The listing builds one solid part. Answer for the finished solid, in the listing's coordinates (mm). Face numbers are marked on the shaded views. Round coordinates to 2 decimals unless told otherwise and drop trailing zeros. Write each loop counter-clockwise with the first axis right and the second up, starting at its lowest first coordinate (ties: lowest second). Pieces come first, ordered by that corner, then holes.
from build123d import *

# Parameters (mm, degrees)
SKETCH1_W           = 80
SKETCH1_H           = 36
BASE_FLANGE1_DEPTH  = 1.5
SKETCH6_W           = 70
SKETCH6_H           = 24
BOSS_EXTRUDE1_DEPTH = 7
SKETCH7_W           = 65
SKETCH7_H           = 15
CUT_EXTRUDE1_DEPTH  = 0.5
CUT_EXTRUDE2_DEPTH  = 0.5
CUT_EXTRUDE3_REACH  = 46.679
SKETCH9_R           = 1.5
SKETCH10_W          = 48
SKETCH10_H          = 2
BOSS_EXTRUDE2_DEPTH = 2
SKETCH11_W          = 0.5
SKETCH11_H          = 0.5
BOSS_EXTRUDE3_DEPTH = 12
LPATTERN1_COUNT     = 19
LPATTERN1_PITCH     = 2.5


# Sheet-metal steps are written as plain solids
with BuildPart() as part:
    # Sketch1 → Base-Flange1 (new body)
    with BuildSketch(Plane.XY):
        Rectangle(SKETCH1_W, SKETCH1_H)
    extrude(amount=-BASE_FLANGE1_DEPTH)

    # Sketch6 → Boss-Extrude1 (add)
    with BuildSketch(Plane.XY):
        Rectangle(SKETCH6_W, SKETCH6_H)
    extrude(amount=BOSS_EXTRUDE1_DEPTH)

    # Sketch7 → Cut-Extrude1 (cut)
    with BuildSketch(Plane.XY.offset(7)):
        Rectangle(SKETCH7_W, SKETCH7_H)
    extrude(amount=-CUT_EXTRUDE1_DEPTH, mode=Mode.SUBTRACT)

    # Sketch8 → Cut-Extrude2 (cut)
    with BuildSketch(Plane.XY.offset(7)):
        with BuildLine():
            Line((32, 9.25), (-32, 9.25))
            ThreePointArc((-32, 9.25), (-32.5, 9.75), (-32, 10.25))
            Line((-32, 10.25), (32, 10.25))
            ThreePointArc((32, 10.25), (32.5, 9.75), (32, 9.25))
        make_face()
        with BuildLine():
            Line((32, -9.25), (-32, -9.25))
            ThreePointArc((-32, -9.25), (-32.5, -9.75), (-32, -10.25))
            Line((-32, -10.25), (32, -10.25))
            ThreePointArc((32, -10.25), (32.5, -9.75), (32, -9.25))
        make_face()
    extrude(amount=-CUT_EXTRUDE2_DEPTH, mode=Mode.SUBTRACT)

    # Sketch9 → Cut-Extrude3 (cut, up to next)
    with BuildSketch(Plane(origin=(0, 0, -1.5), x_dir=(-1, 0, 0), z_dir=(0, 0, -1)), mode=Mode.PRIVATE) as cut_extrude3_sk1:
        with Locations((-37.5, 15.5)):
            Circle(SKETCH9_R)
    cut_extrude3_tool1 = extrude(cut_extrude3_sk1.sketch, amount=-CUT_EXTRUDE3_REACH, mode=Mode.PRIVATE) & part.part
    # Sketch9 → Cut-Extrude3 (cut, up to next)
    with BuildSketch(Plane(origin=(0, 0, -1.5), x_dir=(-1, 0, 0), z_dir=(0, 0, -1)), mode=Mode.PRIVATE) as cut_extrude3_sk2:
        with Locations((-37.5, -15.5)):
            Circle(SKETCH9_R)
    cut_extrude3_tool2 = extrude(cut_extrude3_sk2.sketch, amount=-CUT_EXTRUDE3_REACH, mode=Mode.PRIVATE) & part.part
    # Sketch9 → Cut-Extrude3 (cut, up to next)
    with BuildSketch(Plane(origin=(0, 0, -1.5), x_dir=(-1, 0, 0), z_dir=(0, 0, -1)), mode=Mode.PRIVATE) as cut_extrude3_sk3:
        with Locations((37.5, 15.5)):
            Circle(SKETCH9_R)
    cut_extrude3_tool3 = extrude(cut_extrude3_sk3.sketch, amount=-CUT_EXTRUDE3_REACH, mode=Mode.PRIVATE) & part.part
    # Sketch9 → Cut-Extrude3 (cut, up to next)
    with BuildSketch(Plane(origin=(0, 0, -1.5), x_dir=(-1, 0, 0), z_dir=(0, 0, -1)), mode=Mode.PRIVATE) as cut_extrude3_sk4:
        with Locations((37.5, -15.5)):
            Circle(SKETCH9_R)
    cut_extrude3_tool4 = extrude(cut_extrude3_sk4.sketch, amount=-CUT_EXTRUDE3_REACH, mode=Mode.PRIVATE) & part.part
    add(cut_extrude3_tool1.solids().sort_by_distance((37.5, 15.5, -1.5))[0], mode=Mode.SUBTRACT)
    add(cut_extrude3_tool2.solids().sort_by_distance((37.5, -15.5, -1.5))[0], mode=Mode.SUBTRACT)
    add(cut_extrude3_tool3.solids().sort_by_distance((-37.5, 15.5, -1.5))[0], mode=Mode.SUBTRACT)
    add(cut_extrude3_tool4.solids().sort_by_distance((-37.5, -15.5, -1.5))[0], mode=Mode.SUBTRACT)

    # Sketch10 → Boss-Extrude2 (add)
    with BuildSketch(Plane(origin=(0, 0, -1.5), x_dir=(-1, 0, 0), z_dir=(0, 0, -1))):
        with Locations((8, 15)):
            Rectangle(SKETCH10_W, SKETCH10_H)
    extrude(amount=BOSS_EXTRUDE2_DEPTH)

    # Sketch11 → Boss-Extrude3 (add)
    with BuildSketch(Plane(origin=(0, 0, -3.5), x_dir=(-1, 0, 0), z_dir=(0, 0, -1))):
        with Locations((30.5, 15)):
            Rectangle(SKETCH11_W, SKETCH11_H)
    boss_extrude3 = extrude(amount=BOSS_EXTRUDE3_DEPTH)

    # LPattern1: Boss-Extrude3 ×19
    with Locations(*[(i * LPATTERN1_PITCH, 0, 0) for i in range(1, LPATTERN1_COUNT)]):
        add(boss_extrude3)


solid = part.part
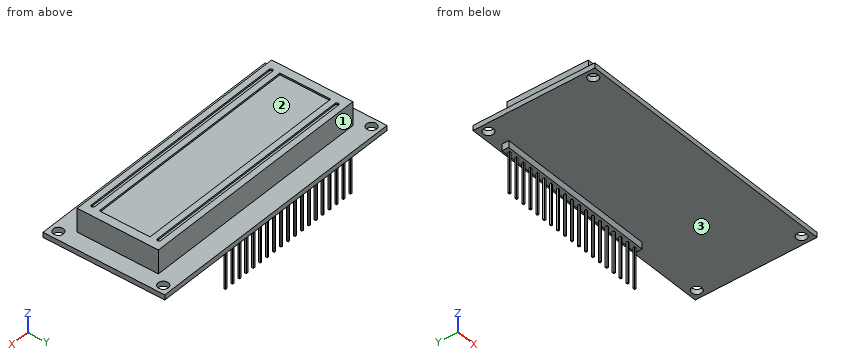
1. Section D-D on z = -5 is taken. Give the number of separate pieces and of enclosed holes in the cut face, plus the area to 3 significant figures.
Geometry says:
separate pieces: 19
enclosed holes: 0
area: 4.75 mm2
2. Straight lines are drawn through the part: line 1 along Y through (x, z) = (-37.5, -0.95); line 2 along X through (y, z) = (-2, 2.75); line 3 along Z through (x, y) = (-32.5, -13.5). For each, find the intervals that lie inside material, in ascending order.
Geometry says:
line 1: y = -18 to -17, -14 to 14, 17 to 18
line 2: x = -35 to 35
line 3: z = -1.5 to 0
3. For a pull along Y with two mould halves and no side action, classify the marked faces 1, 2 and 3 as released by +Y, released by -Y, zero draft, split by the parting line, or undercut.
Geometry says:
face 1: released by +Y
face 2: undercut
face 3: zero draft
4. Given pin 1 (10 mm diameter, centred on x = -5, y = 8.5, fed in from -Z); pin 2 (0.6 mm diameter, centred on y = 14.5, z = -3, fed in from +X); pin 3 (8 mm diameter, centred on x = -10.5, z = -4, fed in from -Y); pin 4 (2 mm diameter, centred on x = 27, z = 2.5, fed in from -Y), each flat-ended and moving along its own axis, determine where each tip first touches the part or whether it passes through.
Geometry says:
pin 1: stops at z = -1.5
pin 2: stops at x = 16
pin 3: stops at y = -18
pin 4: stops at y = -12
5. Section C-C on y = 1 is taken. Determine the outline of the cut face in (x, z).
Geometry says:
outline: (-40, -1.5) - (40, -1.5) - (40, 0) - (35, 0) - (35, 7) - (32.5, 7) - (32.5, 6.5) - (-32.5, 6.5) - (-32.5, 7) - (-35, 7) - (-35, 0) - (-40, 0) - close
6. Section A-A on x = 37.5 is taken. Determine the outline of the cut face in (y, z).
Geometry says:
outline: (-18, -1.5) - (-17, -1.5) - (-17, 0) - (-18, 0) - close; (-14, -1.5) - (14, -1.5) - (14, 0) - (-14, 0) - close; (17, -1.5) - (18, -1.5) - (18, 0) - (17, 0) - close
7. Section B-B on y = -15.5 is taken. Determine the outline of the cut face in (x, z), plus the area to 3 significant figures.
Geometry says:
outline: (-40, -1.5) - (-39, -1.5) - (-39, 0) - (-40, 0) - close; (-36, -1.5) - (36, -1.5) - (36, 0) - (-36, 0) - close; (39, -1.5) - (40, -1.5) - (40, 0) - (39, 0) - close
area: 111 mm2
